Verification items for the finished model (mm, model axes). Round coordinates to 2 decimals unless told otherwise and drop trailing zeros. Order: outer loops, then holes, each group sorted by start corner. A loop starts at its lowest first (then second) coordinate and runs counter-clockwise, first axis right, second up. Notation, with made-up numbers: (-24, -36.75) -> (-1, -36.75) arc R20 cw to (-1, -19.75) -> close; hole circle Ø11 at (33, 14.25). An arc over 180 degrees is marked (long way). Put each result on its own line as item: value.
from build123d import *

# Parameters (mm, degrees)
SKETCH1_W           = 25.4
SKETCH1_H           = 25.4
BOSS_EXTRUDE1_DEPTH = 348.829051578
SKETCH2_R           = 6.35
CUT_EXTRUDE1_DEPTH  = 26.4


with BuildPart() as part:
    # Sketch1 → Boss-Extrude1 (new body)
    with BuildSketch(Plane(origin=(0, 0, 0), x_dir=(0, 0, -1), z_dir=(1, 0, 0))):
        Rectangle(SKETCH1_W, SKETCH1_H)
    extrude(amount=-BOSS_EXTRUDE1_DEPTH)

    # Sketch2 → Cut-Extrude1 (cut, through all)
    with BuildSketch(Plane(origin=(0, 12.7, 0), x_dir=(1, 0, 0), z_dir=(0, 1, 0))):
        with Locations((-336.129051578, 0)):
            Circle(SKETCH2_R)
        with Locations((-12.7, 0)):
            Circle(SKETCH2_R)
    extrude(amount=-CUT_EXTRUDE1_DEPTH, mode=Mode.SUBTRACT)


solid = part.part
Item 1: Gauge pin test, flat ends, axial feed: pin 1 Ø10 at (y, z) = (9.5, 7.5) entering from +X; pin 2 Ø10 at (x, z) = (-12.7, 0) entering from +Y. Record the tip position at first contact, or that the pin passes through.
Check sheet entries:
pin 1: stops at x = 0
pin 2: passes through
Item 2: Section check C-C on y = -7. Record the boundary of the cut face in (x, z).
Check sheet entries:
outline: (-348.83, -12.7) -> (0, -12.7) -> (0, 12.7) -> (-348.83, 12.7) -> close; hole circle Ø12.7 at (-336.13, 0); hole circle Ø12.7 at (-12.7, 0)
Item 3: Material ranges on L1, parallel to X at y = -0.75, z = 0; L2, parallel to X at y = 3.25, z = -0.75; L3, parallel to Z at x = -12.7, y = -1.25, recorded low to high. Write a range as [from, to].
Check sheet entries:
L1: x = [-348.83, -342.48], [-329.78, -19.05], [-6.35, 0]
L2: x = [-348.83, -342.43], [-329.82, -19.01], [-6.39, 0]
L3: z = [-12.7, -6.35], [6.35, 12.7]
Item 4: Section check A-A on x = -12.7. Record the boundary of the cut face in (y, z), then the cut area to 3 significant figures.
Check sheet entries:
outline: (-12.7, -12.7) -> (12.7, -12.7) -> (12.7, -6.35) -> (-12.7, -6.35) -> close; (-12.7, 6.35) -> (12.7, 6.35) -> (12.7, 12.7) -> (-12.7, 12.7) -> close
area: 323 mm^2
Item 5: Section check B-B on z = 0. Record the boundary of the cut face in (x, y).
Check sheet entries:
outline: (-348.83, -12.7) -> (-342.48, -12.7) -> (-342.48, 12.7) -> (-348.83, 12.7) -> close; (-329.78, -12.7) -> (-19.05, -12.7) -> (-19.05, 12.7) -> (-329.78, 12.7) -> close; (-6.35, -12.7) -> (0, -12.7) -> (0, 12.7) -> (-6.35, 12.7) -> close
Item 6: Release check for a two-part mould opening along X. For faces 1 (the cylindrical face through (-6.643, 0.178, -1.907)), 2 (the flat face through (-172, -12.7, 0)), 3 (the flat face through (-348.829, 0, 0)), 4 (the cylindrical face through (-342.473, 0.178, -0.279)) record: +X half, -X half, draft (parallel to the pull), parting line (faces both ways), or undercut.
Check sheet entries:
face 1: undercut
face 2: draft
face 3: -X half
face 4: undercut
